Autodesk Inventor part; units mm, degrees
ref_plane "YZ Plane" through (0, 0, 0) normal (1, 0, 0) x (0, 1, 0)
ref_plane "XZ Plane" through (0, 0, 0) normal (0, 1, 0) x (-1, 0, 0)
ref_plane "XY Plane" through (0, 0, 0) normal (0, 0, 1) x (1, 0, 0)
sketch "Sketch1" plane through (0, 0, 0) normal (0, 0, 1) x (1, 0, 0)
  line L0 (8, 60) -> (32, 60)
  line L1 (32, -60) -> (8, -60)
  line L2 (0, -52) -> (0, 52)
  line L3 (40, 20) -> (142, 20)
  line L4 (150, 12) -> (150, -12)
  line L5 (142, -20) -> (40, -20)
  line L6 (40, 52) -> (40, 20)
  line L7 (40, -20) -> (40, -52)
  line L8 (0, 0) -> (150, 0) construction
  arc A0 (8, 60) -> (0, 52) centre (8, 52) ccw
  arc A1 (0, -52) -> (8, -60) centre (8, -52) ccw
  arc A2 (40, 52) -> (32, 60) centre (32, 52) ccw
  arc A3 (142, -20) -> (150, -12) centre (142, -12) ccw
  arc A4 (150, 12) -> (142, 20) centre (142, 12) ccw
  arc A5 (32, -60) -> (40, -52) centre (32, -52) ccw
  point P0 (0, 0)
  point P1 (40, -60)
  point P2 (0, -60)
  point P3 (150, -20)
  point P4 (150, 20)
  dimension "d0" = 40
  dimension "d1" = 40
  dimension "d2" = 150
  dimension "d3" = 8
  dimension "d4" = 8
  dimension "d5" = 120
extrude "Extrusion1" add sketch "Sketch1" along normal blind 5
sketch "Sketch2" plane through (0, 0, 5) normal (0, 0, 1) x (1, 0, 0)
  line L0 (150, -12) -> (150, 12)
  line L1 (40, -20) -> (142, -20)
  point P0 (0, 0)
  point P1 (142.5, 0)
  dimension "d8" = 7.5
  dimension "d9" = 20
hole "Hole1" at (142.5, 0, 5) direction (0, 0, -1) diameter 7 end through all
sketch "Sketch3" plane through (0, 0, 5) normal (0, 0, 1) x (1, 0, 0)
  line L0 (0, 52) -> (0, -52)
  point P0 (0, 0)
  point P1 (20, 0)
  dimension "d17" = 20
hole "Hole2" at (20, 0, 5) direction (0, 0, -1) diameter 2 depth 1
properties part number "PistonBC" material "MDF Medium Density Fiberboard"
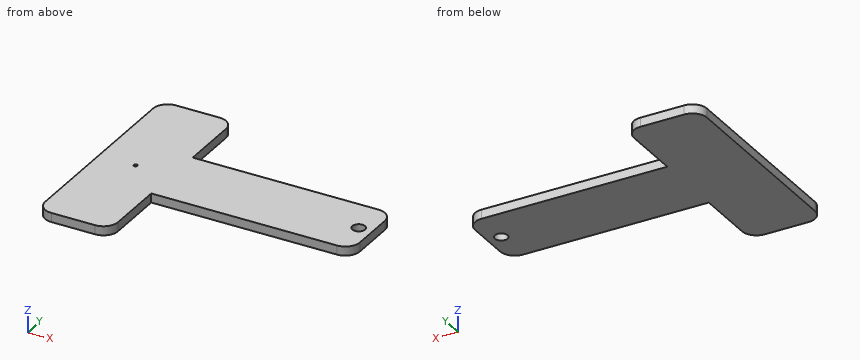
Design review of the part built by this model. Coordinates are the model's own, in mm. Round coordinates to 2 decimals unless told otherwise and drop trailing zeros. Loops run counter-clockwise (first coordinate to the right, second up) from the corner with the lowest first, then second, coordinate; pieces in that order, holes last. Notation, with made-up numbers: M 57,46 L 94,46 A27 cw 94,63 Z; hole C -4.75,59.25 d10. An arc over 180 degrees is marked long. Answer as a JSON object with one key per item and string values.
Item 1: We need section B-B on y = -46.5. Give the boundary of the cut face in (x, z), and give its area (3 significant figures).
Answer sheet:
{"outline": "M 0,0 L 40,0 L 40,5 L 0,5 Z", "area": "200 mm^2"}
Item 2: We need section C-C on x = 108. Give the boundary of the cut face in (y, z), and give its area (3 significant figures).
Answer sheet:
{"outline": "M -20,0 L 20,0 L 20,5 L -20,5 Z", "area": "200 mm^2"}
Item 3: Wall thickness on L1, parallel to X at y = 0, z = 4.3; L2, parallel to Y at x = 142.5, z = 2.05; L3, parallel to X at y = 0, z = 1.75: over which ranges is each line inside the solid? List them lowest first. Write a range as from..to.
Answer sheet:
{"L1": "x = 0..19, 21..139, 146..150", "L2": "y = -19.98..-3.5, 3.5..19.98", "L3": "x = 0..139, 146..150"}
Item 4: We need section A-A on z = 2.3. Give the boundary of the cut face in (x, y).
Answer sheet:
{"outline": "M 0,-52 A8 ccw 8,-60 L 32,-60 A8 ccw 40,-52 L 40,-20 L 142,-20 A8 ccw 150,-12 L 150,12 A8 ccw 142,20 L 40,20 L 40,52 A8 ccw 32,60 L 8,60 A8 ccw 0,52 Z; hole C 142.5,0 d7"}
Item 5: Clearance check with flat-ended pins moving along their axes: P1, Ø1, axis at x = 36.5, z = 2.5, coming from the +Y side; P2, Ø0.6, axis at x = 20, y = 0, coming from the +Z side; P3, Ø1, axis at y = 19, z = 1, coming from the +X side. State where each tip first meets the part, or that it passes through.
Answer sheet:
{"P1": "stops at y = 58.93", "P2": "stops at z = 4", "P3": "stops at x = 146.66"}
